Model file for the job. Use its own axes, mm. A direction names the side the tool comes from. Round coordinates to 2 decimals unless told otherwise and drop trailing zeros. Order: outer loops, then holes, each group sorted by start corner. A loop starts at its lowest first (then second) coordinate and runs counter-clockwise, first axis right, second up. Notation, with made-up numbers: (15, -31) - (23, -31) arc R29 ccw to (23, -10) - close; hole circle Ø4 at (53.25, -18.5). An arc over 180 degrees is marked (long way). Use one line per item in the form item = value.
from build123d import *

# Parameters (mm, degrees)
SKETCH_1_W          = 51
SKETCH_1_H          = 26.2
EXTRUDE_1_DEPTH     = 1.5
SKETCH_2_R          = 4.9
SKETCH_2_R_2        = 7.4
SKETCH_2_W          = 7.6
SKETCH_2_H          = 9.8
SKETCH_2_W_2        = 4.1
SKETCH_2_H_2        = 9.5
SKETCH_2_W_3        = 9.5
EXTRUDE_2_DEPTH     = 9.5
SKETCH_3_R          = 1.05
CUT_EXTRUDE_2_DEPTH = 31.201158918


with BuildPart() as part:
    # Эскиз1 → Бобышка-Вытянуть1 (new body)
    with BuildSketch(Plane.XY):
        Rectangle(SKETCH_1_W, SKETCH_1_H)
    extrude(amount=EXTRUDE_1_DEPTH)

    # Эскиз2 → Бобышка-Вытянуть2 (add)
    with BuildSketch(Plane.XY.offset(1.5)):
        with Locations((17.845463421, 7.569209816)):
            Circle(SKETCH_2_R)
        with Locations((-1.340380905, 5.519215491)):
            Circle(SKETCH_2_R_2)
        with Locations((-16.5, -7.1)):
            Circle(SKETCH_2_R)
        with Locations((-21.2, 4.2)):
            Rectangle(SKETCH_2_W, SKETCH_2_H)
        with Locations((21.2, -4.2)):
            Rectangle(SKETCH_2_W, SKETCH_2_H)
        with Locations((-8.15, -7.85)):
            Rectangle(SKETCH_2_W_2, SKETCH_2_H_2)
        with Locations((-3.565582746, -7.85)):
            Rectangle(SKETCH_2_W_2, SKETCH_2_H_2)
        with Locations((5.669869249, -7.851273466)):
            Rectangle(SKETCH_2_W_3, SKETCH_2_H_2)
    extrude(amount=EXTRUDE_2_DEPTH)

    # Эскиз3 → Вырез-Вытянуть2 (cut, through all)
    with BuildSketch(Plane.XY.offset(1.5)):
        with Locations((-24.200212884, 11.79290343)):
            Circle(SKETCH_3_R)
        with Locations((24.199787116, 11.79290343)):
            Circle(SKETCH_3_R)
        with Locations((24.199787116, -11.70709657)):
            Circle(SKETCH_3_R)
        with Locations((-24.200212884, -11.70709657)):
            Circle(SKETCH_3_R)
    extrude(amount=-CUT_EXTRUDE_2_DEPTH, mode=Mode.SUBTRACT)


solid = part.part
(1) Slice it at B-B on x = -16.5. Give the cut face in (y, z).
Report:
outline = (-13.1, 0) - (13.1, 0) - (13.1, 1.5) - (-2.2, 1.5) - (-2.2, 11) - (-12, 11) - (-12, 1.5) - (-13.1, 1.5) - close
(2) Slice it at D-D on y = -4. Give the cut face in (x, z), then the cut area to 3 significant figures.
Report:
outline = (-25.5, 0) - (25.5, 0) - (25.5, 1.5) - (25, 1.5) - (25, 11) - (17.4, 11) - (17.4, 1.5) - (10.42, 1.5) - (10.42, 11) - (0.92, 11) - (0.92, 1.5) - (-1.52, 1.5) - (-1.52, 11) - (-5.62, 11) - (-5.62, 1.5) - (-6.1, 1.5) - (-6.1, 11) - (-10.2, 11) - (-10.2, 1.5) - (-12.71, 1.5) - (-12.71, 11) - (-20.29, 11) - (-20.29, 1.5) - (-25.5, 1.5) - close
area = 389 mm2
(3) Pin check, flat tips, straight feed: pin 1 (3 mm diameter, centred on y = -6, z = 4.5, fed in from -X); pin 2 (1.7 mm diameter, centred on x = -24.2, y = 11.79, fed in from +Z); pin 3 (2 mm diameter, centred on y = -8, z = 6.5, fed in from +X); pin 4 (5 mm diameter, centred on y = 6.5, z = 5.5, fed in from +X). Stop position of each tip, or through.
Report:
pin_1 = -21.4
pin_2 = through
pin_3 = 25
pin_4 = 22.75
(4) Tool access for faces 5 (the face through (0.92, -8, 6)), 6 (the face through (6, -12.601, 6)), 7 (the face through (10.42, -8, 6)), 8 (the face through (-21, 9.1, 6)), 9 (the face through (-8, -3.1, 6)): list every direction of +Z, -Z, +X, -X, +Y, -Y with a clear straight run to the whole face (end or side of a thin tool).
Report:
face_5 = +Z, -Y
face_6 = +Z, +X, -X, -Y
face_7 = +Z, +Y, -Y
face_8 = +Z, -X, +Y
face_9 = +Z
(5) Slice it at C-C on y = -8. Give the cut face in (x, z), then the cut area to 3 significant figures.
Report:
outline = (-25.5, 0) - (25.5, 0) - (25.5, 1.5) - (25, 1.5) - (25, 11) - (17.4, 11) - (17.4, 1.5) - (10.42, 1.5) - (10.42, 11) - (0.92, 11) - (0.92, 1.5) - (-1.52, 1.5) - (-1.52, 11) - (-5.62, 11) - (-5.62, 1.5) - (-6.1, 1.5) - (-6.1, 11) - (-10.2, 11) - (-10.2, 1.5) - (-11.68, 1.5) - (-11.68, 11) - (-21.32, 11) - (-21.32, 1.5) - (-25.5, 1.5) - close
area = 408 mm2
(6) Slice it at A-A on z = 10.25. Give the cut face in (x, y).
Report:
outline = (-25, -0.7) - (-17.4, -0.7) - (-17.4, 9.1) - (-25, 9.1) - close; circle Ø9.8 at (-16.5, -7.1); (-10.2, -12.6) - (-6.1, -12.6) - (-6.1, -3.1) - (-10.2, -3.1) - close; circle Ø14.8 at (-1.34, 5.52); (-5.62, -12.6) - (-1.52, -12.6) - (-1.52, -3.1) - (-5.62, -3.1) - close; (0.92, -12.6) - (10.42, -12.6) - (10.42, -3.1) - (0.92, -3.1) - close; circle Ø9.8 at (17.85, 7.57); (17.4, -9.1) - (25, -9.1) - (25, 0.7) - (17.4, 0.7) - close
(7) Probe probe 1 along X at (y, z) = (-4.5, 4); probe 2 along X at (y, z) = (5.5, 4.75); probe 3 along X at (y, z) = (-4.25, 9). List the from-to ranges inside material, lowest first. Write a range as [from, to].
Report:
probe_1 = [-20.65, -12.35], [-10.2, -6.1], [-5.62, -1.52], [0.92, 10.42], [17.4, 25]
probe_2 = [-25, -17.4], [-8.74, 6.06], [13.4, 22.29]
probe_3 = [-20.49, -12.51], [-10.2, -6.1], [-5.62, -1.52], [0.92, 10.42], [17.4, 25]
(8) Pull direction X, two halves, no side cores. Call faces 1 (the face through (0, -3, 1.5)), 2 (the face through (25.5, 0, 1)), 3 (the face through (21, -4, 11)), 4 (the face through (-25.5, 0, 1)): released by +X, released by -X, zero draft, split by the parting line, or undercut.
Report:
face_1 = undercut
face_2 = released by +X
face_3 = zero draft
face_4 = released by -X
